Input: part model. Units: mm. Frame: model coordinates. A direction names the side the tool comes from. Give positions to 0.01 mm unless a question says otherwise; leave off trailing zeros. Loops run counter-clockwise (first coordinate to the right, second up) from the corner with the lowest first, then second, coordinate; pieces in that order, holes last. Notation, with made-up numbers: (44.5, -37) -> (93.5, -37) arc R17 ccw to (93.5, -24) -> close; hole circle Ø1 at (-16, 71). An arc over 180 degrees is marked (long way). Use CSV: the item, a comma, the result in double quotes.
```python
from build123d import *

# Parameters (mm, degrees)
BOSS_EXTRUDE1_DEPTH      = 25
BOSS_EXTRUDE1_DEPTH_BACK = 1.0186
SKETCH1_W                = 50
SKETCH1_H                = 50
SKETCH11_R               = 5
CUT_EXTRUDE17_DEPTH      = 15
SKETCH14_R               = 5
CUT_EXTRUDE18_DEPTH      = 25


with BuildPart() as part:
    # Sketch1 → Boss-Extrude1 (new, two sides: drawn at the far end of the back side and taken through both)
    with BuildSketch(Plane(origin=(0, 0, 0), x_dir=(1, 0, 0), z_dir=(0, 1, 0)).offset(-BOSS_EXTRUDE1_DEPTH_BACK)):
        Rectangle(SKETCH1_W, SKETCH1_H)
    extrude(amount=BOSS_EXTRUDE1_DEPTH + BOSS_EXTRUDE1_DEPTH_BACK)

    # Sketch10 → Cut-Revolve2 (revolve, cut)
    with BuildSketch(Plane.XY):
        with BuildLine():
            Line((-5, 10), (5, 10))
            ThreePointArc((5, 10), (0, 15), (-5, 10))
        make_face()
    revolve(axis=Axis((-5, 10, 0), (1, 0, 0)), mode=Mode.SUBTRACT)

    # Sketch11 → Cut-Extrude17 (cut)
    with BuildSketch(Plane(origin=(0, 25, 0), x_dir=(1, 0, 0), z_dir=(0, 1, 0))):
        with Locations(Location((0, 0, 0), (0, 0, 270))):
            Circle(SKETCH11_R)
    extrude(amount=-CUT_EXTRUDE17_DEPTH, mode=Mode.SUBTRACT)

    # Sketch14 → Cut-Extrude18 (cut)
    with BuildSketch(Plane.XY.offset(25)):
        with Locations((0, 10)):
            Circle(SKETCH14_R)
    extrude(amount=-CUT_EXTRUDE18_DEPTH, mode=Mode.SUBTRACT)


solid = part.part
```
1) Mould query, pull axis Z, two halves, no side actions, for faces 1 (the cylindrical face through (0, 18, -5)), 2 (the flat face through (-25, 12, 0)), 3 (the flat face through (0, 12, -25)), 4 (the flat face through (-6, 12, 25)). Classes: pulls with the +Z half, pulls with the -Z half, needs draft (parallel to the pull), parting line crosses it, or undercut.
From the geometry:
face 1,"undercut"
face 2,"needs draft"
face 3,"pulls with the -Z half"
face 4,"pulls with the +Z half"
2) Section query A-A (x = 0). Return loops of the section in (y, z).
From the geometry:
outline,"(-1.02, -25) -> (25, -25) -> (25, -5) -> (10, -5) arc R5 cw to (5, 0) -> (5, 25) -> (-1.02, 25) -> close; (15, 5) -> (25, 5) -> (25, 25) -> (15, 25) -> close"
3) Section query B-B (y = 22.5). Return loops of the section in (x, z).
From the geometry:
outline,"(-25, -25) -> (25, -25) -> (25, 25) -> (-25, 25) -> close; hole circle Ø10 at (0, 0)"
4) Ray query, line 1 (X direction, y = 10, z = 12.75); line 2 (Y direction, x = 0, z = 17). Return the intervals inside material, ascending.
From the geometry:
line 1,"x = -25 to -5, 5 to 25"
line 2,"y = -1.02 to 5, 15 to 25"
5) Reachability of faces 5 (the flat face through (0, 25, -6)), 6 (the cylindrical face through (-1.08, 5.12, 12.68)) from +Z, -Z, +X, -X, +Y, -Y: full face, straight path, thin tool, end or side. Return the list, or none.
From the geometry:
face 5,"+Z, -Z, +X, -X, +Y"
face 6,"+Z"
6) Section query C-C (y = 7.75). Return loops of the section in (x, z), then the cut area to 3 significant figures.
From the geometry:
outline,"(-25, -25) -> (25, -25) -> (25, 25) -> (4.47, 25) -> (4.47, 0) arc R4.47 cw to (-4.47, 0) -> (-4.47, 25) -> (-25, 25) -> close"
area,"2,250 mm^2"
